Design review of the part shown in the three views and the two pictorial views. Dimensions are in mm from the part's minimum x, y and z. Coordinates: 2 decimals unless noted, no trailing zeros. Loops run counter-clockwise (first coordinate to the right, second up) from the corner with the lowest first, then second, coordinate; pieces in that order, holes last. Notation, with made-up numbers: (-12, 33) - (-8, 33) arc R16 ccw to (-8, 58) - close; hole circle Ø1 at (68, 14.5). An arc over 180 degrees is marked (long way). One line per item, written item: value. Start each with the question number.
1. To check wall thickness, follow line 1 (Z direction, x = 29, y = 2.4) (1 decimal); line 2 (Z direction, x = 7, y = 2.85) (1 decimal); line 3 (Z direction, x = 11.5, y = 1.15) (1 decimal). State the ranges of each line that lie inside material, in increasing order. Write a range as from..to.
2. Take a section at A-A, the plane x = 25.5. State the section outline as (y, z) points (1 decimal).
3. Take a section at C-C, the plane z = 18.5. State the section outline as (x, y) points.
4. Insertion check: pin 1 (2 mm diameter, centred on y = 4, z = 23.5, fed in from +X); pin 2 (2 mm diameter, centred on y = 1.5, z = 35, fed in from -X). Each pin has a flat end and moves straight along its axis. Give the tip position at first contact, or say it passes through.
5. The part is to be moulded in two halves that separate along X. For the marked faces 1, 2 and 3, say which applies: released by +X, released by -X, zero draft, split by the parting line, or undercut.
6. Take a section at D-D, the plane x = 36. State the section outline as (y, z) points.
7. Take a section at B-B, the plane y = 3.65. Count the separate pieces of the cut face and the enclosed holes in it, and give its area (3 significant figures).
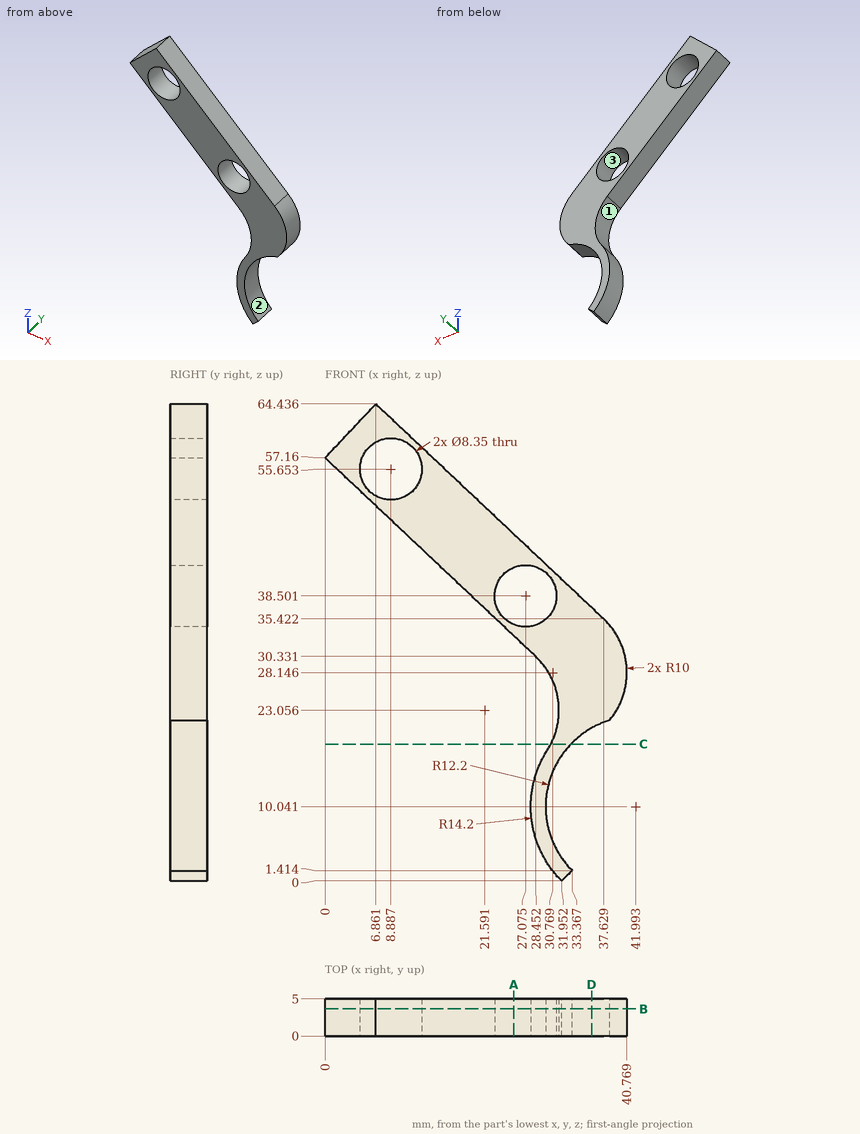
Solutions:
1. line 1: 4.3..15.8, 29.8..34.8, 42.2..43.6
1. line 2: 50.6..51.9, 59.4..64.3
1. line 3: 46.3..52.4, 58.9..60.1
2. outline: (0, 33.1) - (5, 33.1) - (5, 34.6) - (0, 34.6) - close; (0, 42.4) - (5, 42.4) - (5, 46.9) - (0, 46.9) - close
3. outline: (30.49, 0) - (33.2, 0) - (33.2, 5) - (30.49, 5) - close
4. pin 1: x = 40.08
4. pin 2: x = 22.44
5. face 1: released by -X
5. face 2: released by +X
5. face 3: undercut
6. outline: (0, 20.67) - (5, 20.67) - (5, 36.96) - (0, 36.96) - close
7. separate pieces: 1
7. enclosed holes: 2
7. area: 464 mm2
